Verification items for this drawing (mm, ordinates from the low corner). Round coordinates to 2 decimals unless told otherwise and drop trailing zeros. Write each loop counter-clockwise with the first axis right and the second up, starting at its lowest first coordinate (ties: lowest second). Pieces come first, ordered by that corner, then holes.
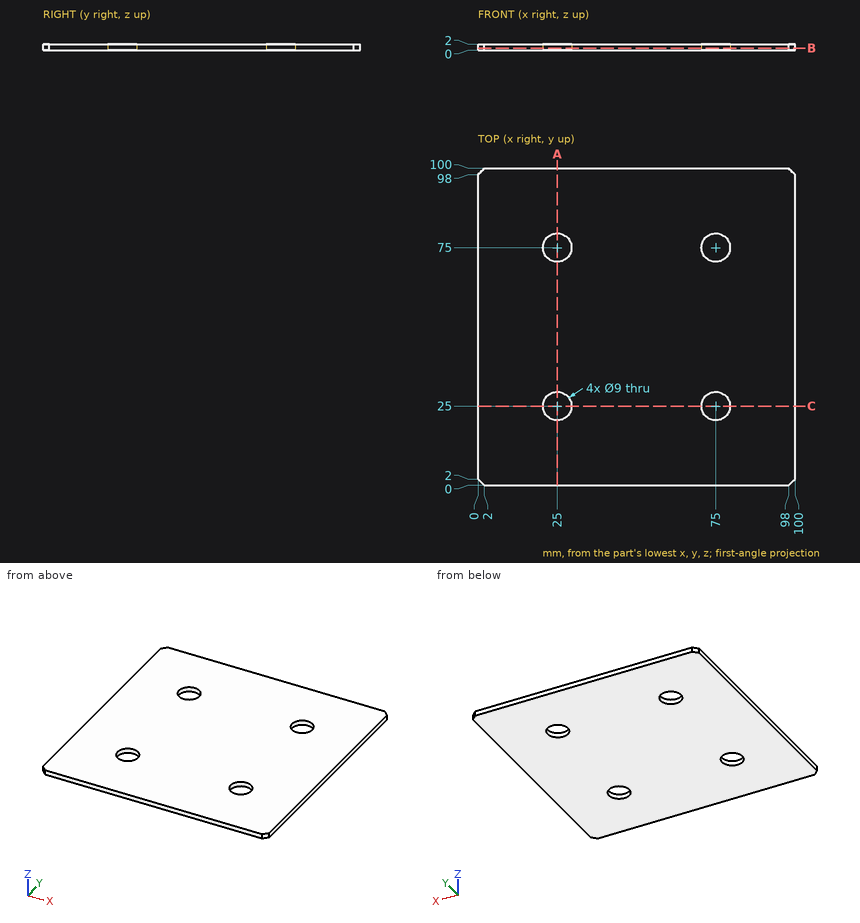
1. Section check A-A (x = 25). Record the cut outline in (y, z), plus the area to 3 significant figures.
2. Depth check by flat-ended pin: pin 1 Ø6 at (x, y) = (61, 53.5) entering from -Z; pin 2 Ø8 at (x, y) = (25, 75) entering from +Z. Enter the tip coordinate at first touch or a pass-through.
3. Section check B-B (z = 0.7). Record the cut outline in (x, y).
4. Scan lines: line 1 along Y through (x, z) = (75, 1.45); line 2 along X through (y, z) = (24.5, 0.9); line 3 along Y through (x, z) = (79, 0.5). Record each from-to range of solid material in increasing order.
Results below:
1. outline: (0, 0) - (20.5, 0) - (20.5, 2) - (0, 2) - close; (29.5, 0) - (70.5, 0) - (70.5, 2) - (29.5, 2) - close; (79.5, 0) - (100, 0) - (100, 2) - (79.5, 2) - close
1. area: 164 mm2
2. pin 1: stops at z = 0
2. pin 2: passes through
3. outline: (0, 2) - (2, 0) - (98, 0) - (100, 2) - (100, 98) - (98, 100) - (2, 100) - (0, 98) - close; hole circle Ø9 at (25, 25); hole circle Ø9 at (25, 75); hole circle Ø9 at (75, 25); hole circle Ø9 at (75, 75)
4. line 1: y = 0 to 20.5, 29.5 to 70.5, 79.5 to 100
4. line 2: x = 0 to 20.53, 29.47 to 70.53, 79.47 to 100
4. line 3: y = 0 to 22.94, 27.06 to 72.94, 77.06 to 100
